from build123d import *

# Parameters (mm, degrees)
BOSS_EXTRUDE1_DEPTH      = 60
BOSS_EXTRUDE2_DEPTH      = 2
BOSS_EXTRUDE3_START      = 60
BOSS_EXTRUDE3_DEPTH      = 2
FILLET1_R                = 5
BOSS_EXTRUDE4_DEPTH      = 2
FILLET2_R                = 2
BOSS_EXTRUDE5_DEPTH      = 2
BOSS_EXTRUDE5_DEPTH_BACK = 1
CHAMFER3_SIZE            = 1
BOSS_EXTRUDE6_DEPTH      = 1
FILLET3_R                = 1
CHAMFER4_SIZE            = 1
CHAMFER4_SIZE_2          = 1.804047755
CUT_EXTRUDE1_DEPTH       = 72.17056976
CUT_EXTRUDE1_DEPTH_BACK  = 72.17056976
SKETCH6_W                = 3.5
SKETCH6_H                = 39


# Some blends are built 0.0001 mm under size
with BuildPart() as part:
    # Sketch1 → Boss-Extrude1 (new body)
    with BuildSketch(Plane.XY):
        with BuildLine():
            Line((-12.5, 0), (12.5, 0))
            ThreePointArc((12.5, 0), (16.035533906, -1.464466094), (17.5, -5))
            Line((17.5, -5), (17.5, -10))
            Line((17.5, -10), (19.5, -10))
            Line((19.5, -10), (19.5, -5))
            ThreePointArc((19.5, -5), (17.449747468, -0.050252532), (12.5, 2))
            Line((12.5, 2), (-12.5, 2))
            ThreePointArc((-12.5, 2), (-17.449747468, -0.050252532), (-19.5, -5))
            Line((-19.5, -5), (-19.5, -10))
            Line((-19.5, -10), (-17.5, -10))
            Line((-17.5, -10), (-17.5, -5))
            ThreePointArc((-17.5, -5), (-16.035533906, -1.464466094), (-12.5, 0))
        make_face()
    extrude(amount=BOSS_EXTRUDE1_DEPTH)

    # Sketch2 → Boss-Extrude2 (add)
    with BuildSketch(Plane.XY):
        with BuildLine():
            Line((19.5, -10), (19.5, -5))
            ThreePointArc((19.5, -5), (17.449747468, -0.050252532), (12.5, 2))
            Line((12.5, 2), (-12.5, 2))
            ThreePointArc((-12.5, 2), (-17.449747468, -0.050252532), (-19.5, -5))
            Line((-19.5, -5), (-19.5, -10))
            Line((-19.5, -10), (19.5, -10))
        make_face()
    extrude(amount=BOSS_EXTRUDE2_DEPTH)

    # Sketch2<2> → Boss-Extrude3 (add)
    with BuildSketch(Plane.XY.offset(BOSS_EXTRUDE3_START)):
        with BuildLine():
            Line((19.5, -10), (19.5, -5))
            ThreePointArc((19.5, -5), (17.449747468, -0.050252532), (12.5, 2))
            Line((12.5, 2), (-12.5, 2))
            ThreePointArc((-12.5, 2), (-17.449747468, -0.050252532), (-19.5, -5))
            Line((-19.5, -5), (-19.5, -10))
            Line((-19.5, -10), (19.5, -10))
        make_face()
    extrude(amount=BOSS_EXTRUDE3_DEPTH)

    # Fillet1
    fillet1_edges = [part.edges().sort_by_distance(p)[0] for p in [
        (-17.5, -7.5, 60),
        (-16.035533906, -1.464466094, 60),
        (0, 0, 60),
        (16.035533906, -1.464466094, 60),
        (-17.449747468, -0.050252532, 62),
        (17.449747468, -0.050252532, 62),
        (-19.5, -7.5, 62),
        (19.5, -7.5, 62),
        (0, 2, 62),
        (17.5, -7.5, 60),
    ]]
    fillet(fillet1_edges, radius=FILLET1_R)

    # Sketch3 → Boss-Extrude4 (add)
    with BuildSketch(Plane.XZ.offset(10)):
        Polygon((-7, 0), (-7, -60), (0, -67), (7, -60), (7, 0), align=None)
    extrude(amount=-BOSS_EXTRUDE4_DEPTH)

    # Fillet2
    fillet2_edges = [part.edges().sort_by_distance(p)[0] for p in [
        (0, -8, 0),
        (-7, -9, 0),
        (7, -9, 0),
    ]]
    fillet(fillet2_edges, radius=FILLET2_R)

    # Sketch4 → Boss-Extrude5 (add, two sides: drawn at the far end of the back side and taken through both)
    with BuildSketch(Plane.XZ.offset(10).offset(-BOSS_EXTRUDE5_DEPTH_BACK)):
        with BuildLine():
            Line((-17.5, 2), (17.5, 2))
            Line((17.5, 2), (17.5, 55))
            ThreePointArc((17.5, 55), (16.035533906, 58.535533906), (12.5, 60))
            Line((12.5, 60), (-12.5, 60))
            ThreePointArc((-12.5, 60), (-16.035533906, 58.535533906), (-17.5, 55))
            Line((-17.5, 55), (-17.5, 2))
        make_face()
        with BuildLine():
            Line((-16.5, 3), (16.5, 3))
            Line((16.5, 3), (16.5, 55))
            ThreePointArc((16.5, 55), (15.328427125, 57.828427125), (12.5, 59))
            Line((12.5, 59), (-12.5, 59))
            ThreePointArc((-12.5, 59), (-15.328427125, 57.828427125), (-16.5, 55))
            Line((-16.5, 55), (-16.5, 3))
        make_face(mode=Mode.SUBTRACT)
    extrude(amount=BOSS_EXTRUDE5_DEPTH + BOSS_EXTRUDE5_DEPTH_BACK)

    # Chamfer3
    chamfer3_edges = [part.edges().sort_by_distance(p)[0] for p in [
        (-17.5, -9, 28.5),
        (-16.035533906, -9, 58.535533906),
        (0, -9, 60),
        (16.035533906, -9, 58.535533906),
        (17.5, -9, 28.5),
        (0, -9, 2),
    ]]
    chamfer(chamfer3_edges, length=CHAMFER3_SIZE - 0.0001)  # a hair under: the kernel refuses the full size

    # Sketch5 → Boss-Extrude6 (add)
    with BuildSketch(Plane(origin=(0, -8, 0), x_dir=(1, 0, 0), z_dir=(0, 1, 0))):
        Polygon((-4.825973992, 0), (-2.477626604, 0), (-2.477626604, 64.522373396), (-4.825973992, 62.174026008), align=None)
        Polygon((4.825973992, 0), (4.825973992, 62.174026008), (2.477626604, 64.522373396), (2.477626604, 0), align=None)
    extrude(amount=BOSS_EXTRUDE6_DEPTH)

    # Fillet3
    fillet3_edges = [part.edges().sort_by_distance(p)[0] for p in [
        (4.825973992, -7, -31.2209876),
        (2.477626604, -7, -32.395161294),
        (-2.477626604, -7, -32.395161294),
        (-4.825973992, -7, -31.2209876),
    ]]
    fillet(fillet3_edges, radius=FILLET3_R - 0.0001)  # a hair under: the kernel refuses the full size

    # Chamfer4
    # the kernel refuses this chamfer: 1.804047755, 1 mm, written as the material it takes off along each edge
    with BuildSketch(Plane(origin=(-0.176240013, -7, -66.823759987), x_dir=(-0.04304000526140607, -0.9981458389905735, -0.043040005261406056), z_dir=(-0.7071067811865475, 0, 0.7071067811865477)), Plane(origin=(7.127360583, -7, -59.872639417), x_dir=(0.043040005261406056, -0.9981458389905735, -0.04304000526140604), z_dir=(-0.7071067811865475, 0, -0.7071067811865477))) as chamfer4_piece_1:
        Polygon((CHAMFER4_SIZE * 0.998145838991, CHAMFER4_SIZE * 0.0608677591653), (-CHAMFER4_SIZE_2 * 0.0608677591744, CHAMFER4_SIZE_2 * 0.998145839141), (0, 0), align=None)
    extrude(amount=9.830368984, mode=Mode.SUBTRACT)

    # Sketch6 → Cut-Extrude1 (cut, two sides: drawn at the far end of the back side and taken through both)
    with BuildSketch(Plane(origin=(0, 2, 0), x_dir=(1, 0, 0), z_dir=(0, 1, 0)).offset(-CUT_EXTRUDE1_DEPTH_BACK)):
        with Locations((12.75, -32.5)):
            Rectangle(SKETCH6_W, SKETCH6_H)
        with Locations((-12.75, -32.5)):
            Rectangle(SKETCH6_W, SKETCH6_H)
    extrude(amount=CUT_EXTRUDE1_DEPTH + CUT_EXTRUDE1_DEPTH_BACK, mode=Mode.SUBTRACT)


solid = part.part
Geometry check sheet. Reference: the model listing, model coordinates, mm. A direction names the side the tool comes from. Give positions to 0.01 mm unless a question says otherwise; leave off trailing zeros.
1. Sectioned sample at B-B (z = 42.5). State how many separate pieces and enclosed holes the cut face has, then the cut area to 3 significant figures.
Completed:
separate pieces: 3
enclosed holes: 0
area: 101 mm2
2. Scan lines: line 1 (X direction, y = -7.5, z = 20); line 2 (X direction, y = -9.5, z = 24.5); line 3 (Z direction, x = -6.5, y = -7.25). Record each from-to range of solid material in increasing order.
Completed:
line 1: x = -19.5 to -17.5, 17.5 to 19.5
line 2: x = -19.5 to -16.5, 16.5 to 19.5
line 3: z = -0.44 to 2, 60 to 62
3. Draft check along X on faces 5 (the face through (3.684, -7.507, -62.058)), 6 (the face through (16.5, -10, 29)), 7 (the face through (-18.07, -7.54, 60.5)). Enter one of: pulls with the +X half, pulls with the -X half, needs draft (parallel to the pull), parting line crosses it, or undercut.
Completed:
face 5: pulls with the +X half
face 6: undercut
face 7: pulls with the -X half
4. Access from +Z, -Z, +X, -X, +Y, -Y to the whole of each face (thin tool, end or side, straight path). Record for faces 1 (the face through (0, -10, 59)), 2 (the face through (13, 1, 52)), 3 (the face through (-6, -8, -32)), 4 (the face through (-15.496, -8.715, 58.063)).
Completed:
face 1: -Y
face 2: +Y, -Y
face 3: -Z, -X, +Y
face 4: none
5. Depth check by flat-ended pin: pin 1 (0.7 mm diameter, centred on x = 12.5, y = 0.5, fed in from +Z); pin 2 (0.7 mm diameter, centred on x = 13, y = 1.5, fed in from -Z); pin 3 (5 mm diameter, centred on x = -8, z = -39, fed in from -Y); pin 4 (8 mm diameter, centred on y = -2, z = -23.5, fed in from +X). Enter the tip coordinate at first touch or a pass-through.
Completed:
pin 1: stops at z = 60.88
pin 2: stops at z = 0
pin 3: stops at y = -10
pin 4: passes through
